Part model, mm, in its own coordinate system. Round coordinates to 2 decimals unless told otherwise and drop trailing zeros. Write each loop counter-clockwise with the first axis right and the second up, starting at its lowest first coordinate (ties: lowest second). Pieces come first, ordered by that corner, then holes. Notation, with made-up numbers: M -38,-13 L -21,-13 A22 ccw -21,-4 Z; hole C 59.25,-34.75 d9. An arc over 180 degrees is marked long. Use a Markdown table: item, result. Add a question column.
1) Slice it at D-D on x = -19. Write the cut outline in (y, z), plus the area to 3 significant figures.
2) Slice it at C-C on z = -5.25. Write the cut outline in (x, y), plus the area to 3 significant figures.
3) Slice it at A-A on z = 0. Write the cut outline in (x, y), plus the area to 3 significant figures.
4) Wall check: probe 1 along Y at (x, z) = (-7, -4.5); probe 2 along X at (y, z) = (-32.5, -1.75); probe 3 along X at (y, z) = (-12.5, 4.5). Give the ranges that are in metal, low to high.
5) Drop flat-ended pins along their axis: P1, Ø5, axis at y = -18.5, z = -5, coming from the -X side; P2, Ø4, axis at x = 12, z = -2, coming from the -Y side; P3, Ø2, axis at y = 4.5, z = -4.5, coming from the -X side. Give the stop position or say it passes through.
6) Slice it at B-B on x = 10. Write the cut outline in (y, z).
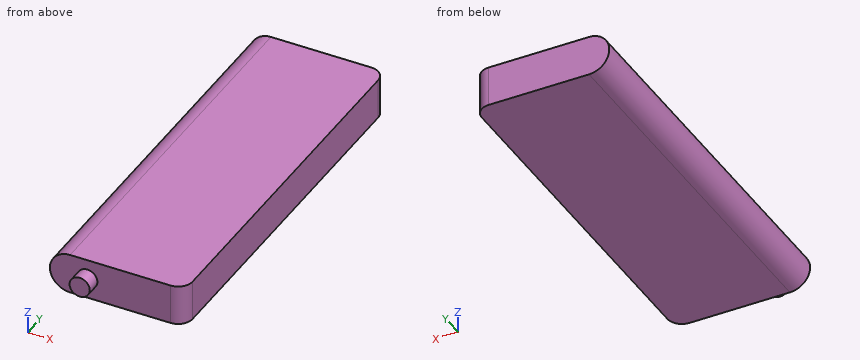
```python
from build123d import *

# Parameters (mm, degrees)
PAD_DEPTH    = 65.75
FILLET_R     = 5
SKETCH001_R  = 3.5
PAD001_DEPTH = 5


with BuildPart() as part:
    # Sketch → Pad (new body, symmetric)
    with BuildSketch(Plane.XZ):
        with BuildLine():
            Line((-16.4, 7), (23.4, 7))
            Line((23.4, 7), (23.4, -7))
            Line((23.4, -7), (-16.4, -7))
            ThreePointArc((-16.4, 7), (-23.4, 0), (-16.4, -7))
        make_face()
    extrude(amount=PAD_DEPTH, both=True)

    # Fillet
    fillet_edges = [part.edges().sort_by_distance(p)[0] for p in [
        (23.4, -65.75, 0),
        (23.4, 65.75, 0),
    ]]
    fillet(fillet_edges, radius=FILLET_R)

    # Sketch001 (on Face6 of Fillet) → Pad001 (join)
    with BuildSketch(Plane.XZ.offset(65.75)):
        with Locations((-10.432093, 0)):
            Circle(SKETCH001_R)
    extrude(amount=PAD001_DEPTH)


solid = part.part
```
Entries:
| question | item | result |
|---|---|---|
| 1 | outline | M -65.75,-6.5 L 65.75,-6.5 L 65.75,6.5 L -65.75,6.5 Z |
| 1 | area | 1,710 mm^2 |
| 2 | outline | M -21.03,-65.75 L 18.4,-65.75 A5 ccw 23.4,-60.75 L 23.4,60.75 A5 ccw 18.4,65.75 L -21.03,65.75 Z |
| 2 | area | 5,830 mm^2 |
| 3 | outline | M -23.4,-65.75 L -13.93,-65.75 L -13.93,-70.75 L -6.93,-70.75 L -6.93,-65.75 L 18.4,-65.75 A5 ccw 23.4,-60.75 L 23.4,60.75 A5 ccw 18.4,65.75 L -23.4,65.75 Z |
| 3 | area | 6,180 mm^2 |
| 4 | probe 1 | y = -65.75 to 65.75 |
| 4 | probe 2 | x = -23.18 to 23.4 |
| 4 | probe 3 | x = -21.76 to 23.4 |
| 5 | P1 | stops at x = -22.94 |
| 5 | P2 | stops at y = -65.75 |
| 5 | P3 | stops at x = -22.46 |
| 6 | outline | M -65.75,-7 L 65.75,-7 L 65.75,7 L -65.75,7 Z |
